Source: CAD feature listing. Evaluate the final solid. Frame: model axes, mm. Face numbers are marked on the shaded views. Give positions to 0.01 mm unless a question says otherwise; leave off trailing zeros. Order: outer loops, then holes, each group sorted by start corner. A loop starts at its lowest first (then second) coordinate and runs counter-clockwise, first axis right, second up. Notation, with made-up numbers: (67.5, -16.75) -> (120.5, -16.75) arc R28 ccw to (120.5, 9.25) -> close; hole circle Ø6 at (41.5, -19). An arc over 180 degrees is marked (long way). Answer in a Markdown table with one row per item.
```python
from build123d import *

# Parameters (mm, degrees)
SKETCH1_R           = 2.000000064
SKETCH1_R_2         = 1.5
BOSS_EXTRUDE1_DEPTH = 3.175


with BuildPart() as part:
    # Sketch1 → Boss-Extrude1 (new body)
    with BuildSketch(Plane(origin=(0, 0, 0), x_dir=(1, 0, 0), z_dir=(0, 1, 0))):
        with BuildLine():
            Line((15.24, -11), (-15.24, -6.35))
            ThreePointArc((-15.24, -6.35), (-21.59, 0), (-15.24, 6.35))
            Line((-15.24, 6.35), (15.24, 11))
            ThreePointArc((15.24, 11), (26.24, 0), (15.24, -11))
        make_face()
        with Locations((-15.24, 0)):
            Circle(SKETCH1_R, mode=Mode.SUBTRACT)
        with Locations((15.24, 0)):
            Circle(SKETCH1_R, mode=Mode.SUBTRACT)
        with Locations((15.24, 8)):
            Circle(SKETCH1_R_2, mode=Mode.SUBTRACT)
        with Locations((23.24, 0)):
            Circle(SKETCH1_R_2, mode=Mode.SUBTRACT)
        with Locations((15.24, -8)):
            Circle(SKETCH1_R_2, mode=Mode.SUBTRACT)
    extrude(amount=BOSS_EXTRUDE1_DEPTH)


solid = part.part
```
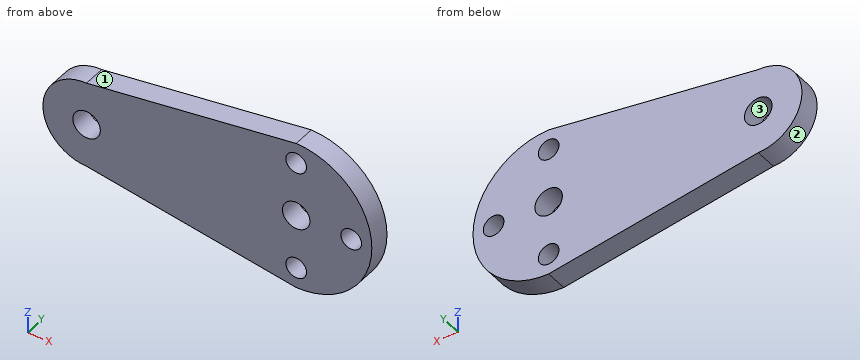
(1) Ray query, probe 1 along X at (y, z) = (1.8, 0); probe 2 along Z at (x, y) = (-15.24, 1.15); probe 3 along X at (y, z) = (2.4, 1). Return the intervals inside material, ascending.
A:
| item | result |
|---|---|
| probe 1 | x = -21.59 to -17.24, -13.24 to 13.24, 17.24 to 21.74, 24.74 to 26.24 |
| probe 2 | z = -6.35 to -2, 2 to 6.35 |
| probe 3 | x = -21.51 to -16.97, -13.51 to 13.51, 16.97 to 22.12, 24.36 to 26.19 |
(2) Pull-direction query (Z, two-part tool) for the marked faces 1, 2 and 3; classes: +Z half, -Z half, draft (parallel to the pull), parting line (faces both ways), or undercut.
A:
| item | result |
|---|---|
| face 1 | +Z half |
| face 2 | parting line |
| face 3 | undercut |
(3) Section query D-D (x = 23.24). Return the cut outline in (y, z) (3 decimals), plus the area to 3 significant figures.
A:
| item | result |
|---|---|
| outline | (0, -7.55) -> (3.175, -7.55) -> (3.175, -1.5) -> (0, -1.5) -> close; (0, 1.5) -> (3.175, 1.5) -> (3.175, 7.55) -> (0, 7.55) -> close |
| area | 38.4 mm^2 |
(4) Section query A-A (z = 0). Return the cut outline in (x, y) (3 decimals).
A:
| item | result |
|---|---|
| outline | (-21.59, 0) -> (-17.24, 0) -> (-17.24, 3.175) -> (-21.59, 3.175) -> close; (-13.24, 0) -> (13.24, 0) -> (13.24, 3.175) -> (-13.24, 3.175) -> close; (17.24, 0) -> (21.74, 0) -> (21.74, 3.175) -> (17.24, 3.175) -> close; (24.74, 0) -> (26.24, 0) -> (26.24, 3.175) -> (24.74, 3.175) -> close |
(5) Section query C-C (z = 8.5). Return the cut outline in (x, y) (3 decimals).
A:
| item | result |
|---|---|
| outline | (-1.147, 0) -> (13.826, 0) -> (13.826, 3.175) -> (-1.147, 3.175) -> close; (16.654, 0) -> (22.222, 0) -> (22.222, 3.175) -> (16.654, 3.175) -> close |
(6) First-contact query: pin 1 Ø8 at (x, z) = (0.5, 1) entering from -Y; pin 2 Ø2.5 at (x, z) = (15.24, 0) entering from +Y. Flat tips, straight axial feed; report the tip coordinate or a pass-through.
A:
| item | result |
|---|---|
| pin 1 | stops at y = 0 |
| pin 2 | passes through |
(7) Section query B-B (y = 2.4). Return the cut outline in (x, z).
A:
| item | result |
|---|---|
| outline | (-15.24, -6.35) -> (15.24, -11) arc R11 ccw to (15.24, 11) -> (-15.24, 6.35) arc R6.35 ccw to start; hole circle Ø4 at (-15.24, 0); hole circle Ø4 at (15.24, 0); hole circle Ø3 at (15.24, -8); hole circle Ø3 at (15.24, 8); hole circle Ø3 at (23.24, 0) |
